Autodesk Inventor part; units mm, degrees
ref_plane "YZ Plane" through (0, 0, 0) normal (1, 0, 0) x (0, 1, 0)
ref_plane "XZ Plane" through (0, 0, 0) normal (0, 1, 0) x (-1, 0, 0)
ref_plane "XY Plane" through (0, 0, 0) normal (0, 0, 1) x (1, 0, 0)
sketch "Sketch1" plane through (0, 0, 0) normal (0, 1, 0) x (-1, 0, 0)
  circle A0 centre (18.5, 28) radius 23.85
  circle A1 centre (37, -23.25) radius 13.85
  arc A2 (-38.7137, -52.0928) -> (-48.6766, -40.9345) centre (-35, -38.75) ccw
  circle A3 centre (-30.9, 25.8) radius 13.85
  circle A4 centre (0, -23.25) radius 13.85
  line L0 (56.25, 58.25) -> (-56.25, 58.25)
  line L1 (-56.25, -58.25) -> (56.25, -58.25)
  line L2 (0, -105.9299) -> (0, 123.2086) construction
  line L3 (-76.4777, -38.75) -> (-5.35, -38.75) construction
  line L4 (-123.5447, -23.25) -> (82.5572, -23.25) construction
  line L5 (56.25, -58.25) -> (56.25, 58.25) construction
  line L6 (56.25, 58.25) -> (-56.25, 58.25)
  line L7 (-56.25, 58.25) -> (-56.25, -41.25)
  line L8 (-39.25, -58.25) -> (56.25, -58.25)
  line L9 (56.25, -58.25) -> (56.25, 58.25)
  line L10 (-56.25, -58.25) -> (-41.25, -58.25)
  line L11 (-41.25, -56.25) -> (-41.25, -54.0196)
  line L12 (-50.6516, -43.25) -> (-54.25, -43.25)
  line L13 (-56.25, -43.25) -> (-56.25, -58.25)
  arc A5 (-41.25, -56.25) -> (-39.25, -58.25) centre (-39.25, -56.25) ccw
  arc A6 (-56.25, -41.25) -> (-54.25, -43.25) centre (-54.25, -41.25) ccw
  arc A7 (-38.7137, -52.0928) -> (-41.25, -54.0196) centre (-39.25, -54.0196) ccw
  arc A8 (-50.6516, -43.25) -> (-48.6766, -40.9345) centre (-50.6516, -41.25) ccw
  point P0 (0, 0)
  point P1 (0, 0)
  point P2 (-48.0986, -43.25)
  point P3 (-56.25, -43.25)
  point P4 (-41.25, -51.1096)
  dimension "d0" = 47.7
  dimension "d1" = 27.7
  dimension "d2" = 27.7
  dimension "d3" = 27.7
  dimension "d4" = 27.7
  dimension "d5" = 116.5
  dimension "d6" = 112.5
  dimension "d7" = 37
  dimension "d8" = 18.5
  dimension "d9" = 30.9
  dimension "d10" = 19.5
  dimension "d11" = 35
  dimension "d12" = 35
  dimension "d13" = 25.8
  dimension "d14" = 28
  dimension "d20" = 112.5
  dimension "d21" = 56.25
  dimension "d22" = 58.25
  dimension "d23" = 116.5
  dimension "d24" = 23.25
  dimension "d25" = 35
  dimension "d26" = 35
  dimension "d27" = 19.25
  dimension "d28" = 37.75
  dimension "d29" = 30.25
  dimension "d30" = 2
  dimension "d31" = 2
  dimension "d32" = 15
  dimension "d33" = 15
  dimension "d34" = 2
extrude "Extrusion1" add sketch "Sketch1" along normal blind 3
sketch "Sketch2" plane through (0, 0, 0) normal (0, -1, 0) x (1, 0, 0)
  line L0 (70.8974, 51.25) -> (-70.9169, 51.25) construction
  line L1 (-56.25, 58.25) -> (56.25, 58.25) construction
  line L2 (56.25, 58.25) -> (56.25, -41.25) construction
  line L3 (-56.25, -58.25) -> (-56.25, 58.25) construction
  point P0 (0, 0)
  point P1 (50.25, 51.25)
  point P2 (-50.25, 51.25)
  dimension "d35" = 7
  dimension "d36" = 6
  dimension "d37" = 6
hole "Hole1" at (50.25, 0, 51.25) at (-50.25, 0, 51.25) direction (0, 1, 0) diameter 5 end through all
sketch "Sketch3" plane through (-56.25, 0, 58.25) normal (0, 0, 1) x (1, 0, 0)
  line L0 (112.5, 0) -> (112.5, 3)
  line L1 (0, 0) -> (112.5, 0)
  line L2 (112.5, 0) -> (112.5, 3)
  line L3 (112.5, 3) -> (0, 3)
  line L4 (0, 3) -> (0, 0)
  point P0 (56.25, 0)
extrude "Extrusion2" cut sketch "Sketch3" against normal blind 0.3
properties part number "Bottle Spacer Base"
Model file for the job. Use its own axes, mm. A direction names the side the tool comes from. Coordinates: 2 decimals unless noted, no trailing zeros. Order: outer loops, then holes, each group sorted by start corner. A loop starts at its lowest first (then second) coordinate and runs counter-clockwise, first axis right, second up. Notation, with made-up numbers: (87, -11.5) -> (100, -11.5) arc R31 cw to (100, 19.5) -> close; hole circle Ø11 at (-30, 21). An arc over 180 degrees is marked (long way). Return JSON: item names as keys, results as strings. Group by question number.
Item 1: Saw through at D-D on x = -37. Write the cut outline in (y, z).
Item 2: Pull direction Z, two halves, no side cores. Call faces 3 (the cylindrical face through (25.01, 1.48, -29.16)), 4 (the flat face through (-1, 2, 57.95)), 5 (the cylindrical face through (-49.29, 1.52, 48.94)), 6 (the flat face through (-56.25, 1, -1)): pulls with the +Z half, pulls with the -Z half, needs draft (parallel to the pull), parting line crosses it, or undercut.
Item 3: Saw through at B-B on x = -17. Write the cut outline in (y, z).
Item 4: Saw through at C-C on y = 1.15. Write the cut outline in (x, z).
Item 5: Saw through at A-A on z = -23.25. Write the cut outline in (x, y).
Item 6: Wall check: line 1 along Z through (x, y) = (3, 2.65); line 2 along Z through (x, y) = (-38, 1.45); line 3 along X through (y, z) = (2.75, -11.5). Give the ranges that are in metal, low to high. Write a range as [from, to].
Item 7: Tool access for faces 1 (the cylindrical face through (17.69, 1.48, 21.64)), 2 (the flat face through (52, 1, -43.25)): list every direction of +Z, -Z, +X, -X, +Y, -Y with a clear straight run to the whole face (end or side of a thin tool).
Values found:
{
 "1": {"outline": "(0, -58.25) -> (3, -58.25) -> (3, -37.1) -> (0, -37.1) -> close; (0, -9.4) -> (3, -9.4) -> (3, 12.95) -> (0, 12.95) -> close; (0, 43.05) -> (3, 43.05) -> (3, 57.95) -> (0, 57.95) -> close"},
 "2": {"face 3": "undercut", "face 4": "pulls with the +Z half", "face 5": "undercut", "face 6": "needs draft"},
 "3": {"outline": "(0, -58.25) -> (3, -58.25) -> (3, 4.2) -> (0, 4.2) -> close; (0, 51.8) -> (3, 51.8) -> (3, 57.95) -> (0, 57.95) -> close"},
 "4": {"outline": "(-56.25, -58.25) -> (39.25, -58.25) arc R2 ccw to (41.25, -56.25) -> (41.25, -54.02) arc R2 ccw to (38.71, -52.09) arc R13.85 cw (long way) to (48.68, -40.93) arc R2 ccw to (50.65, -43.25) -> (54.25, -43.25) arc R2 ccw to (56.25, -41.25) -> (56.25, 57.95) -> (-56.25, 57.95) -> close; hole circle Ø5 at (-50.25, 51.25); hole circle Ø27.7 at (-37, -23.25); hole circle Ø47.7 at (-18.5, 28); hole circle Ø27.7 at (0, -23.25); hole circle Ø27.7 at (30.9, 25.8); hole circle Ø5 at (50.25, 51.25)"},
 "5": {"outline": "(-56.25, 0) -> (-50.85, 0) -> (-50.85, 3) -> (-56.25, 3) -> close; (-23.15, 0) -> (-13.85, 0) -> (-13.85, 3) -> (-23.15, 3) -> close; (13.85, 0) -> (56.25, 0) -> (56.25, 3) -> (13.85, 3) -> close"},
 "6": {"line 1": "z = [-58.25, -36.77], [-9.73, 17.68], [38.32, 57.95]", "line 2": "z = [-58.25, -37.06], [-9.44, 14.27], [41.73, 57.95]", "line 3": "x = [-56.25, -44.33], [-29.67, -7.33], [7.33, 56.25]"},
 "7": {"face 1": "+Y, -Y", "face 2": "-Z, +X, +Y, -Y"}
}
